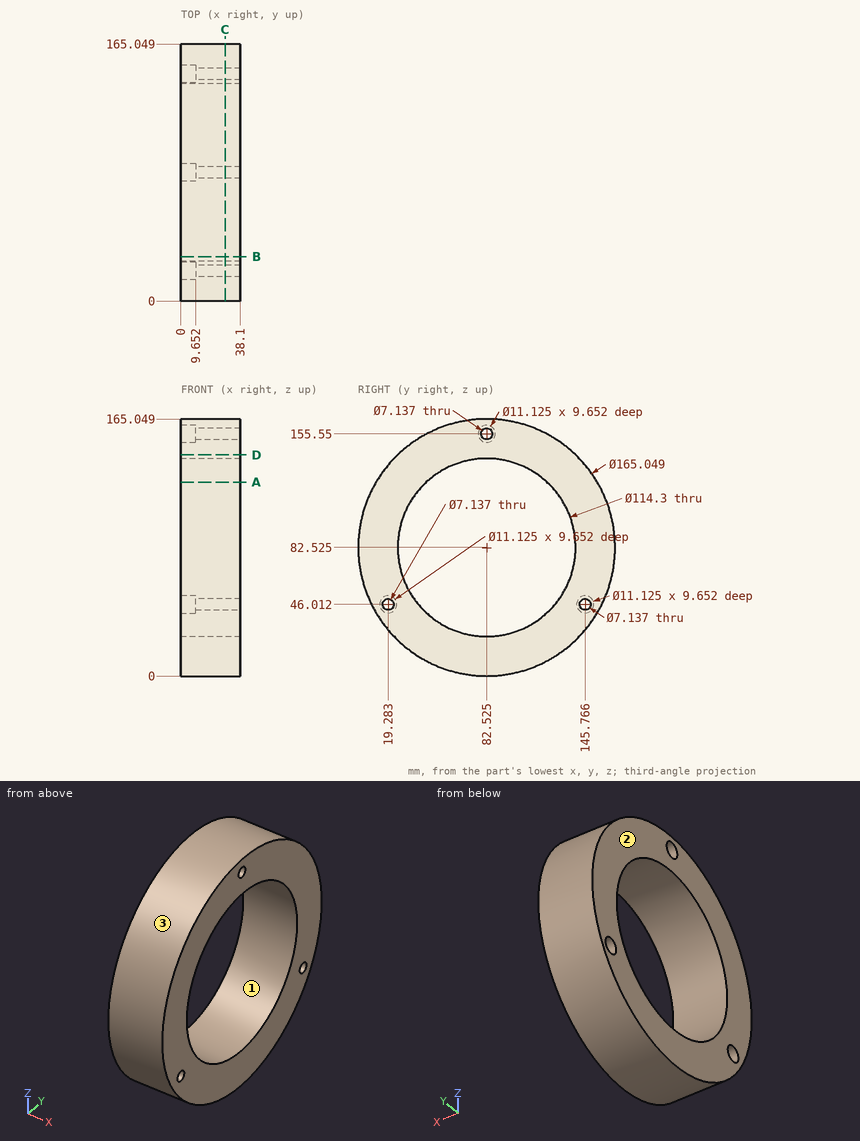
The drawing under review shows one solid part. Ordinate dimensions are in mm from its lowest x, y, z. Coordinates: 2 decimals unless noted, no trailing zeros. Order: outer loops, then holes, each group sorted by start corner. A loop starts at its lowest first (then second) coordinate and runs counter-clockwise, first axis right, second up. Notation, with made-up numbers: (14, 29) -> (50, 29) arc R11 ccw to (50, 45) -> close; hole circle Ø9 at (-24.5, 40.25). An arc over 180 degrees is marked (long way). Answer in a Markdown table with one row per item.
(1) Consider section D-D (z = 142). Write out the cut boundary in (x, y) (1 decimal), plus the area to 3 significant figures.
Answers:
| item | result |
|---|---|
| outline | (0, 25.3) -> (38.1, 25.3) -> (38.1, 139.7) -> (0, 139.7) -> close |
| area | 4,360 mm² |
(2) Consider section C-C (x = 28.5). State how many separate pieces and enclosed holes the cut face has, plus the area to 3 significant figures.
Answers:
| item | result |
|---|---|
| separate pieces | 1 |
| enclosed holes | 4 |
| area | 11,000 mm² |
(3) Insertion check: pin 1 (18 mm diameter, centred on y = 82.52, z = 155.55, fed in from -X); pin 2 (5.5 mm diameter, centred on y = 144, z = 45.5, fed in from -X); pin 3 (1.5 mm diameter, centred on x = 29.5, z = 134.5, fed in from -Y); pin 4 (12 mm diameter, centred on y = 37.5, z = 88.5, fed in from -X). Each pin has a flat end and moves straight along its axis. Give the tip position at first contact, or say it passes through.
Answers:
| item | result |
|---|---|
| pin 1 | x = 0 |
| pin 2 | x = 9.65 |
| pin 3 | y = 17.82 |
| pin 4 | through |
(4) Consider section B-B (y = 28.5). Write out the cut boundary in (x, z) (1 decimal), plus the area to 3 significant figures.
Answers:
| item | result |
|---|---|
| outline | (0, 20.1) -> (38.1, 20.1) -> (38.1, 63.9) -> (0, 63.9) -> close; (0, 101.2) -> (38.1, 101.2) -> (38.1, 144.9) -> (0, 144.9) -> close |
| area | 3,330 mm² |
(5) Consider section A-A (z = 124.5). Write out the cut boundary in (x, y), plus the area to 3 significant figures.
Answers:
| item | result |
|---|---|
| outline | (0, 11.47) -> (38.1, 11.47) -> (38.1, 43.74) -> (0, 43.74) -> close; (0, 121.31) -> (38.1, 121.31) -> (38.1, 153.58) -> (0, 153.58) -> close |
| area | 2,460 mm² |
(6) The part is to be moulded in two halves that separate along Y. For the marked faces 1, 2 and 3, say which applies: +Y half, -Y half, draft (parallel to the pull), parting line (faces both ways), or undercut.
Answers:
| item | result |
|---|---|
| face 1 | undercut |
| face 2 | draft |
| face 3 | parting line |
(7) Wall thickness on line 1 along Z through (x, y) = (31.5, 143) (1 decimal); line 2 along Y through (x, z) = (3.5, 47); line 3 along Z through (x, y) = (13.5, 67) (1 decimal): over which ranges is each line inside the solid? List them lowest first.
Answers:
| item | result |
|---|---|
| line 1 | 26.4 to 43.8, 48.3 to 138.7 |
| line 2 | 8.04 to 13.81, 24.76 to 37.76, 127.29 to 140.29, 151.24 to 157.01 |
| line 3 | 1.5 to 27.5, 137.5 to 163.6 |
